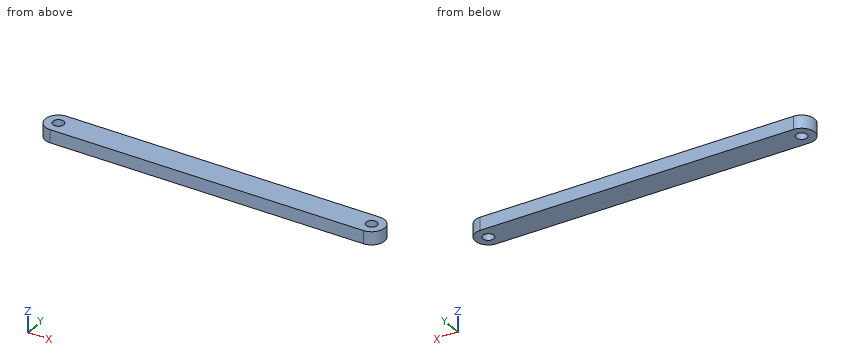
from build123d import *

# Parameters (mm, degrees)
BOSS_EXTRUDE1_DEPTH = 3
SKETCH2_W           = 155.927688531
SKETCH2_H           = 55.200678057
CUT_EXTRUDE1_DEPTH  = 1
SKETCH3_R           = 2.1
CUT_EXTRUDE2_DEPTH  = 66.383484153


with BuildPart() as part:
    # Sketch1 → Boss-Extrude1 (new, symmetric)
    with BuildSketch(Plane.XY):
        with BuildLine():
            Line((60, 5), (-60, 5))
            ThreePointArc((-60, 5), (-65, 0), (-60, -5))
            Line((-60, -5), (60, -5))
            ThreePointArc((60, -5), (65, 0), (60, 5))
        make_face()
    extrude(amount=BOSS_EXTRUDE1_DEPTH, both=True)

    # Sketch2 → Cut-Extrude1 (cut)
    with BuildSketch(Plane.XY.offset(3)):
        with Locations((-0.853618733, 0.071134895)):
            Rectangle(SKETCH2_W, SKETCH2_H)
    extrude(amount=-CUT_EXTRUDE1_DEPTH, mode=Mode.SUBTRACT)

    # Sketch3 → Cut-Extrude2 (cut, through all)
    with BuildSketch(Plane(origin=(0, 0, -3), x_dir=(-1, 0, 0), z_dir=(0, 0, -1))):
        with Locations((-60, 0)):
            Circle(SKETCH3_R)
        with Locations((60, 0)):
            Circle(SKETCH3_R)
    extrude(amount=-CUT_EXTRUDE2_DEPTH, mode=Mode.SUBTRACT)


solid = part.part
For this review, take the finished solid that the model builds, in its own axes (mm). Round coordinates to 2 decimals unless told otherwise and drop trailing zeros. Loops run counter-clockwise (first coordinate to the right, second up) from the corner with the lowest first, then second, coordinate; pieces in that order, holes last. Notation, with made-up numbers: (-36, 51.25) - (-10, 51.25) arc R23 ccw to (-10, 82.25) - close; hole circle Ø3 at (-35.5, 4). An arc over 180 degrees is marked (long way). Put each result on its own line as item: value. Start each with the question number.
1. Consider section A-A on y = 0. State the section outline as (x, z) points, plus the area to 3 significant figures.
2. For probe 1 along Y at (x, z) = (-60, -0.9); probe 2 along X at (y, z) = (-0.75, 1.85); probe 3 along X at (y, z) = (-3, 1.2), list the stretches that pass through material, from the lowest coordinate up. Write a range as [from, to].
3. Consider section B-B on z = 0.25. State the section outline as (x, y) points, plus the area to 3 significant figures.
Result sheet:
1. outline: (-65, -3) - (-62.1, -3) - (-62.1, 2) - (-65, 2) - close; (-57.9, -3) - (57.9, -3) - (57.9, 2) - (-57.9, 2) - close; (62.1, -3) - (65, -3) - (65, 2) - (62.1, 2) - close
1. area: 608 mm^2
2. probe 1: [-5, -2.1], [2.1, 5]
2. probe 2: [-64.94, -61.96], [-58.04, 58.04], [61.96, 64.94]
2. probe 3: [-64, 64]
3. outline: (-60, -5) - (60, -5) arc R5 ccw to (60, 5) - (-60, 5) arc R5 ccw to start; hole circle Ø4.2 at (-60, 0); hole circle Ø4.2 at (60, 0)
3. area: 1,250 mm^2
